For this review, use the dimensioned drawing (mm, ordinates from the lowest corner) and the shaded views. A direction names the side the tool comes from. Give positions to 0.01 mm unless a question says otherwise; leave off trailing zeros. Loops run counter-clockwise (first coordinate to the right, second up) from the corner with the lowest first, then second, coordinate; pieces in that order, holes last. Notation, with made-up numbers: (-36.5, -40) -> (-14.5, -40) arc R19 ccw to (-14.5, -25) -> close; hole circle Ø2 at (60, 0.5). An arc over 180 degrees is marked (long way). Write each question's results on one line, items separated by ' | '. Start each with the question number.
Q1. Insertion check: pin 1 Ø24 at (x, z) = (42, 20.5) entering from +Y; pin 2 Ø1.5 at (x, z) = (44, 21.5) entering from -Y; pin 3 Ø15 at (y, z) = (55, 31.5) entering from +X. Each pin has a flat end and moves straight along its axis. Give the tip position at first contact, or say it passes through.
Q2. We need section D-D (z = 38). Write out the cut boundary in (x, y).
Q3. We need section C-C (x = 22.5). Write out the cut boundary in (y, z), plus the area to 3 significant figures.
Q4. We need section A-A (z = 25). Write out the cut boundary in (x, y), plus the area to 3 significant figures.
Q5. Wall thickness on L1, parallel to Y at x = 41.5, z = 25; L2, parallel to Y at x = 28.5, z = 13; L3, parallel to Z at x = 3, y = 15.5: over which ranges is each line inside the solid? List them lowest first. Write a range as [from, to].
Q6. We need section B-B (y = 15). Write out the cut boundary in (x, z), plus the area to 3 significant figures.
Q7. Mouldability with a two-part tool opening along Z and no side actions: class the marked faces 1, 2 and 3 as released by +Z, released by -Z, zero draft, split by the parting line, or undercut.
Q8. Machinability: for the marked faces 4, 5 and 6, which of the approach directions +Z, -Z, +X, -X, +Y, -Y give a long, thin tool a straight path to every point of the face, cutting with its end or side? Answer none if there is none.
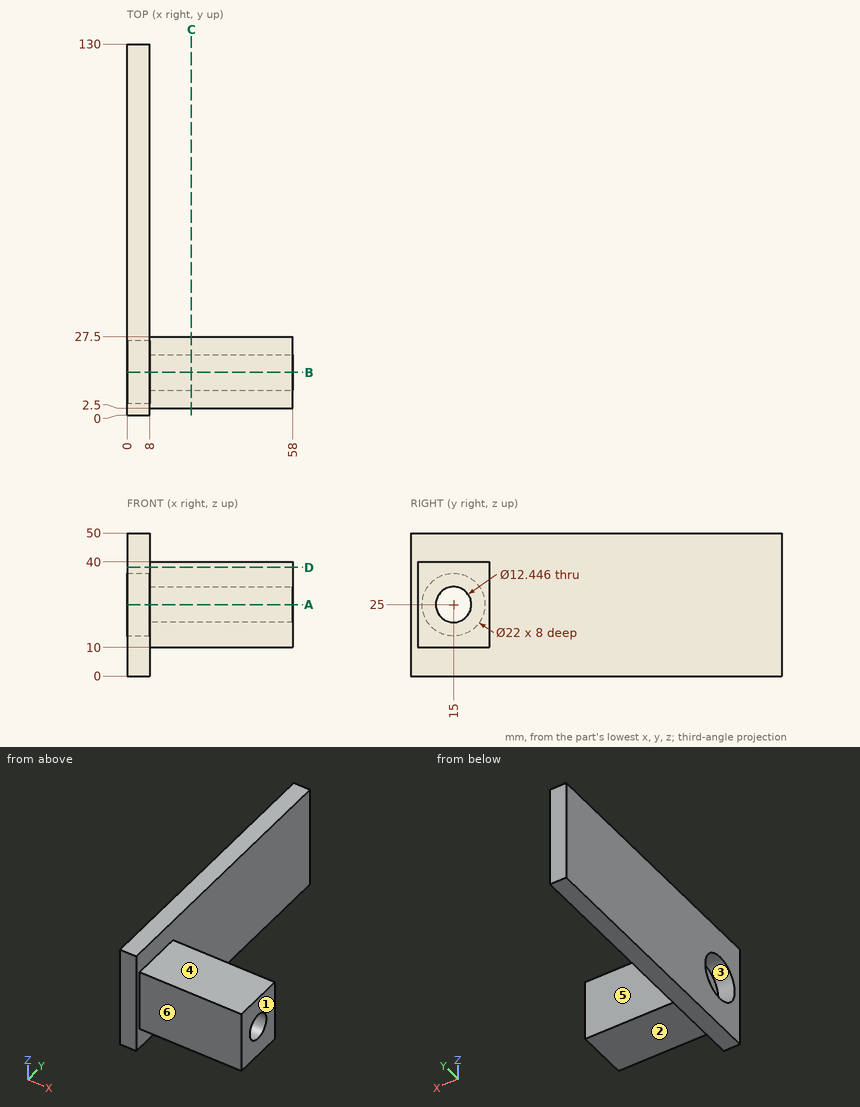
Output:
1) pin 1: y = 27.5 | pin 2: y = 2.5 | pin 3: x = 8
2) outline: (0, 0) -> (8, 0) -> (8, 2.5) -> (58, 2.5) -> (58, 27.5) -> (8, 27.5) -> (8, 130) -> (0, 130) -> close
3) outline: (2.5, 10) -> (27.5, 10) -> (27.5, 40) -> (2.5, 40) -> close; hole circle Ø12.45 at (15, 25) | area: 628 mm2
4) outline: (0, 0) -> (8, 0) -> (8, 2.5) -> (58, 2.5) -> (58, 8.78) -> (8, 8.78) -> (8, 4) -> (0, 4) -> close; (0, 26) -> (8, 26) -> (8, 21.22) -> (58, 21.22) -> (58, 27.5) -> (8, 27.5) -> (8, 130) -> (0, 130) -> close | area: 1,490 mm2
5) L1: [2.5, 8.78], [21.22, 27.5] | L2: [2.5, 27.5] | L3: [0, 14.01], [35.99, 50]
6) outline: (0, 0) -> (8, 0) -> (8, 10) -> (58, 10) -> (58, 18.78) -> (8, 18.78) -> (8, 14) -> (0, 14) -> close; (0, 36) -> (8, 36) -> (8, 31.22) -> (58, 31.22) -> (58, 40) -> (8, 40) -> (8, 50) -> (0, 50) -> close | area: 1,100 mm2
7) face 1: zero draft | face 2: released by -Z | face 3: undercut
8) face 4: +Z, +X, +Y, -Y | face 5: +Z, -Z, +X, +Y | face 6: +Z, -Z, +X, -Y
